from build123d import *

# Parameters (mm, degrees)
CUT_EXTRUDE_1_DEPTH = 5
CUT_EXTRUDE_2_DEPTH = 10


with BuildPart() as part:
    # 草图1 → 旋转1 (revolve)
    with BuildSketch(Plane(origin=(0, 0, 0), x_dir=(1, 0, 0), z_dir=(0, 1, 0))):
        Polygon((12, 50), (0, 50), (0, 20), (19.8, 20), align=None)
        Polygon((19.8, 20), (0, 20), (0, 0), (25, 0), align=None)
    revolve(axis=Axis((0, 0, 0), (0, 0, -1)))

    # 草图2 → 切除-拉伸1 (cut)
    with BuildSketch(Plane(origin=(0, 0, -50), x_dir=(-1, 0, 0), z_dir=(0, 0, -1))):
        Polygon((0, 6.92820323), (-6, 3.464101615), (-6, -3.464101615), (0, -6.92820323), (6, -3.464101615), (6, 3.464101615), align=None)
    extrude(amount=-CUT_EXTRUDE_1_DEPTH, mode=Mode.SUBTRACT)

    # 草图3 → 切除-拉伸2 (cut)
    with BuildSketch(Plane.XY):
        Polygon((0, 15), (-12.990381057, 7.5), (-12.990381057, -7.5), (0, -15), (12.990381057, -7.5), (12.990381057, 7.5), align=None)
    extrude(amount=-CUT_EXTRUDE_2_DEPTH, mode=Mode.SUBTRACT)


solid = part.part
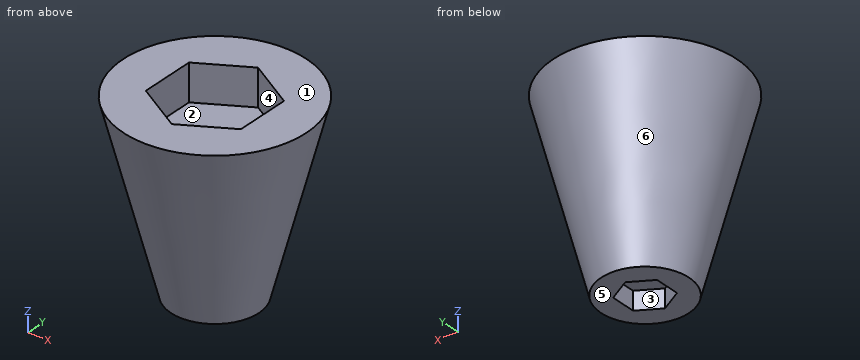
Can you work these out from the model? Positions are in its coordinate system, mm. Face numbers are marked on the shaded views. A direction names the side the tool comes from. Give positions to 0.01 mm unless a question says otherwise; leave off trailing zeros. Loops run counter-clockwise (first coordinate to the right, second up) from the corner with the lowest first, then second, coordinate; pieces in that order, holes last. Notation, with made-up numbers: (76, -26) - (96, -26) arc R24 cw to (96, 5) - close; hole circle Ø2 at (72.25, 44). An arc over 180 degrees is marked (long way). Return JSON: item names as keys, results as strings.
1. I'm going to push flat-ended pins straight in: pin 1 Ø5.5 at (y, z) = (0, -47) entering from +X (3 decimals); pin 2 Ø8 at (y, z) = (3.5, -5.5) entering from -X; pin 3 Ø12 at (x, z) = (-7.5, -24) entering from +Y; pin 4 Ø9.5 at (x, y) = (-1, -2.5) entering from -Z. Where does each tip first touch, or does it pass through?
Output values:
{"pin 1": "stops at x = 13.495", "pin 2": "stops at x = -24.45", "pin 3": "stops at y = 19.62", "pin 4": "stops at z = -50"}
2. I want a section at B-B on z = -38.5. Please give me the cut outline in (x, y), and give its area (3 significant figures).
Output values:
{"outline": "circle Ø29.98 at (0, 0)", "area": "706 mm²"}
3. I want a section at A-A on y = 0. Please give me the cut outline in (x, z), and give its area (3 significant figures).
Output values:
{"outline": "(-25, 0) - (-12, -50) - (-6, -50) - (-6, -45) - (6, -45) - (6, -50) - (12, -50) - (25, 0) - (12.99, 0) - (12.99, -10) - (-12.99, -10) - (-12.99, 0) - close", "area": "1,530 mm²"}
4. We'd pull the mould along Y, two halves only. Please class the marked faces 4, 5 and 6: +Y half, -Y half, draft (parallel to the pull), parting line (faces both ways), or undercut.
Output values:
{"face 4": "undercut", "face 5": "draft", "face 6": "parting line"}
5. If I drill on line 1 (Y direction, x = -8, z = -9.5); line 2 (Y direction, x = 5, z = -3); line 3 (X direction, y = -3, z = -5.5), over which ranges is the centre line in solid material (lowest first)?
Output values:
{"line 1": "y = -21.06 to -10.38, 10.38 to 21.06", "line 2": "y = -23.7 to -12.11, 12.11 to 23.7", "line 3": "x = -23.38 to -12.99, 12.99 to 23.38"}
6. For the marked faces 1, 2 and 3, which set-ups out of +Z, -Z, +X, -X, +Y, -Y let a thin tool reach every point of the face, with its end or its side?
Output values:
{"face 1": "+Z, +X, -X, +Y, -Y", "face 2": "+Z", "face 3": "-Z"}
